Check sheet for the modelled part. Datum: model origin and axes. Units: mm. Face numbers are marked on the shaded views. A direction names the side the tool comes from. Give positions to 0.01 mm unless a question says otherwise; leave off trailing zeros. Write each loop counter-clockwise with the first axis right and the second up, starting at its lowest first coordinate (ties: lowest second). Pieces come first, ordered by that corner, then holes. Notation, with made-up numbers: M 23,74 L 58,74 A28 cw 58,102 Z; hole C 25,33.25 d1. An arc over 180 degrees is marked long. Write item = value, one per line. Start each with the question number.
1) Scan lines: L1, parallel to Z at x = -0.5, y = -1.25; L2, parallel to Y at x = 3.25, z = 1.5; L3, parallel to Z at x = 0, y = 0.5. Record each from-to range of solid material in increasing order.
2) Draft check along Y on the marked faces 4, 5 and 6. Enter one of: pulls with the +Y half, pulls with the -Y half, needs draft (parallel to the pull), parting line crosses it, or undercut.
3) Set-up check for the marked faces 1, 2 and 3: record each of +Z, -Z, +X, -X, +Y, -Y from which the full face is reachable in a straight line by a thin tool's end or side.
4) Sectioned sample at C-C, the plane z = -1.75. Record the cut outline in (x, y), then the cut area to 3 significant figures.
5) Gauge pin test, flat ends, axial feed: pin 1 (1.6 mm diameter, centred on x = -1.5, y = -1.5, fed in from -Z); pin 2 (0.7 mm diameter, centred on x = 2, y = 0.5, fed in from -Z); pin 3 (1.6 mm diameter, centred on x = -1.5, y = -1.5, fed in from +Z). Record the tip position at first contact, or that the pin passes through.
6) Sectioned sample at B-B, the plane y = 3.75. Record the cut outline in (x, z).
7) Sectioned sample at A-A, the plane x = 0. Record the cut outline in (y, z), then the cut area to 3 significant figures.
8) Sectioned sample at D-D, the plane z = 3. Record the cut outline in (x, y).
from build123d import *

# Parameters (mm, degrees)
F0_R     = 2.85
F1_DEPTH = 4
F2_R     = 3.7
F2_R_2   = 2.85
F3_DEPTH = 1.6
F4_R     = 3.7
F4_R_2   = 2.85
F5_DEPTH = 1.6
F7_DEPTH = 8.001
F9_DEPTH = 12.5


with BuildPart() as f1:
    # F0 (on Front) → F1 (new body, symmetric)
    with BuildSketch(Plane.XZ):
        Circle(F0_R)
    extrude(amount=F1_DEPTH, both=True)

    # F2 (on face) → F3 (join)
    with BuildSketch(Plane.XZ.offset(4)):
        Circle(F2_R)
        Circle(F2_R_2, mode=Mode.SUBTRACT)
    extrude(amount=-F3_DEPTH)

    # F4 (on face) → F5 (join)
    with BuildSketch(Plane(origin=(0, 4, 0), x_dir=(-1, 0, 0), z_dir=(0, 1, 0))):
        Circle(F4_R)
        Circle(F4_R_2, mode=Mode.SUBTRACT)
    extrude(amount=-F5_DEPTH)

    # F6 (on face) → F7 (cut, through all)
    with BuildSketch(Plane.XZ.offset(4)):
        with BuildLine():
            ThreePointArc((2.331309, -0.9), (2.45672, -0.457745), (2.499, 0))
            ThreePointArc((2.499, 0), (2.45672, 0.457745), (2.331309, 0.9))
            Line((2.331309, 0.9), (0.9, 0.9))
            Line((0.9, 0.9), (0.9, 2.331309))
            ThreePointArc((0.9, 2.331309), (0, 2.499), (-0.9, 2.331309))
            Line((-0.9, 2.331309), (-0.9, 0.9))
            Line((-0.9, 0.9), (-2.331309, 0.9))
            ThreePointArc((-2.331309, 0.9), (-2.499, 0), (-2.331309, -0.9))
            Line((-2.331309, -0.9), (-0.9, -0.9))
            Line((-0.9, -0.9), (-0.9, -2.331309))
            ThreePointArc((-0.9, -2.331309), (0, -2.499), (0.9, -2.331309))
            Line((0.9, -2.331309), (0.9, -0.9))
            Line((0.9, -0.9), (2.331309, -0.9))
        make_face()
    extrude(amount=-F7_DEPTH, mode=Mode.SUBTRACT)

    # F8 (on Right) → F9 (cut, symmetric)
    with BuildSketch(Plane.YZ):
        with BuildLine():
            Line((1.5, 0), (0, 0))
            Line((0, 0), (-1.5, 0))
            Line((-1.5, 0), (-2, 0))
            ThreePointArc((-2, 0), (-1.853553, -0.353553), (-1.5, -0.5))
            Line((-1.5, -0.5), (1.5, -0.5))
            ThreePointArc((1.5, -0.5), (1.853553, -0.353553), (2, 0))
            Line((2, 0), (1.5, 0))
        make_face()
        with BuildLine():
            Line((0, 0.5), (0, 0))
            Line((0, 0), (1.5, 0))
            Line((1.5, 0), (2, 0))
            ThreePointArc((2, 0), (1.853553, 0.353553), (1.5, 0.5))
            Line((1.5, 0.5), (0, 0.5))
        make_face()
        with BuildLine():
            Line((-1.5, 0), (0, 0))
            Line((0, 0), (0, 0.5))
            Line((0, 0.5), (-1.5, 0.5))
            ThreePointArc((-1.5, 0.5), (-1.853553, 0.353553), (-2, 0))
            Line((-2, 0), (-1.5, 0))
        make_face()
    extrude(amount=F9_DEPTH, both=True, mode=Mode.SUBTRACT)


solid = f1.part
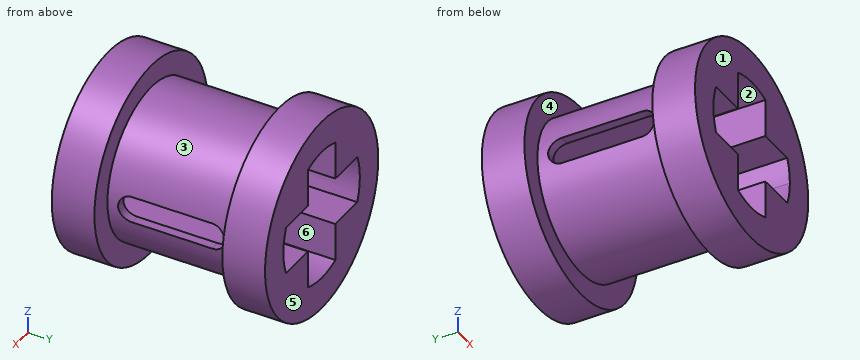
Data:
q1.L1 = -2.81 to -2.45, 2.45 to 2.81
q1.L2 = -4 to -2.4, 2.4 to 4
q1.L3 = -2.85 to -2.5, 2.5 to 2.85
q2.face_4 = undercut
q2.face_5 = pulls with the +Y half
q2.face_6 = needs draft
q3.face_1 = +Z, -Z, +X, -X, -Y
q3.face_2 = +Y, -Y
q3.face_3 = none
q4.outline = M -3.26,-4 L -0.9,-4 L -0.9,4 L -3.26,4 L -3.26,2.4 L -2.25,2.4 L -2.25,-2.4 L -3.26,-2.4 Z; M 0.9,-4 L 3.26,-4 L 3.26,-2.4 L 2.25,-2.4 L 2.25,2.4 L 3.26,2.4 L 3.26,4 L 0.9,4 Z
q4.area = 28.1 mm2
q5.pin_1 = -2.76
q5.pin_2 = -2.32
q5.pin_3 = 2.76
q6.outline = C 0,0 d7.4; hole M -2.33,-0.9 L -0.9,-0.9 L -0.9,-2.33 A2.5 ccw 0.9,-2.33 L 0.9,-0.9 L 2.33,-0.9 A2.5 ccw 2.5,0 A2.5 ccw 2.33,0.9 L 0.9,0.9 L 0.9,2.33 A2.5 ccw -0.9,2.33 L -0.9,0.9 L -2.33,0.9 A2.5 ccw Z
q7.outline = M -4,-3.7 L -2.4,-3.7 L -2.4,-2.85 L 2.4,-2.85 L 2.4,-3.7 L 4,-3.7 L 4,-2.5 L -4,-2.5 Z; M -4,2.5 L 4,2.5 L 4,3.7 L 2.4,3.7 L 2.4,2.85 L -2.4,2.85 L -2.4,3.7 L -4,3.7 Z
q7.area = 11.1 mm2
q8.outline = M -2.17,-4 L 2.17,-4 L 2.17,-2.4 L -2.17,-2.4 Z; M -2.17,2.4 L 2.17,2.4 L 2.17,4 L -2.17,4 Z
